```python
from build123d import *

# Parameters (mm, degrees)
SKETCH_1_R          = 4
SKETCH_1_R_2        = 1.5
EXTRUDE_1_DEPTH     = 2
EXTRUDE_2_DEPTH     = 52
EXTRUDE_START       = 2
SKETCH_3_R          = 4
SKETCH_3_R_2        = 1.5
EXTRUDE_3_DEPTH     = 2
FILLET_1_R          = 3
FILLET_2_R          = 1
SKETCH_4_R          = 4
SKETCH_4_R_2        = 1.5
CUT_EXTRUDE_1_DEPTH = 2
SKETCH_5_R          = 1.5
CUT_EXTRUDE_2_DEPTH = 2


with BuildPart() as part:
    # 草图1 → 凸台-拉伸1 (new body)
    with BuildSketch(Plane.XY):
        with BuildLine():
            Line((8.838834765, -8.838834765), (39.597979746, 21.920310217))
            Line((39.597979746, 21.920310217), (4.242640687, 21.920310217))
            Line((4.242640687, 21.920310217), (-8.838834765, 8.838834765))
            ThreePointArc((-8.838834765, 8.838834765), (-8.838834765, -8.838834765), (8.838834765, -8.838834765))
        make_face()
        Circle(SKETCH_1_R, mode=Mode.SUBTRACT)
        with Locations((4.949747468, -4.949747468)):
            Circle(SKETCH_1_R_2, mode=Mode.SUBTRACT)
        with Locations((-4.949747468, -4.949747468)):
            Circle(SKETCH_1_R_2, mode=Mode.SUBTRACT)
        with Locations((-4.949747468, 4.949747468)):
            Circle(SKETCH_1_R_2, mode=Mode.SUBTRACT)
        with Locations((4.949747468, 4.949747468)):
            Circle(SKETCH_1_R_2, mode=Mode.SUBTRACT)
    extrude(amount=EXTRUDE_1_DEPTH)

    # 草图2 → 凸台-拉伸2 (add)
    with BuildSketch(Plane(origin=(0, 0, 0), x_dir=(-1, 0, 0), z_dir=(0, 0, -1))):
        Polygon((-39.597979746, 21.920310217), (-4.242640687, 21.920310217), (-2.242640687, 19.920310217), (-37.597979746, 19.920310217), align=None)
    extrude(amount=EXTRUDE_2_DEPTH)

    # 草图3 → 凸台-拉伸3 (add)
    with BuildSketch(Plane(origin=(0, 0, -52), x_dir=(-1, 0, 0), z_dir=(0, 0, -1)).offset(EXTRUDE_START)):
        with BuildLine():
            Line((-2.242640687, 19.920310217), (-4.242640687, 21.920310217))
            Line((-4.242640687, 21.920310217), (-39.597979746, 21.920310217))
            Line((-39.597979746, 21.920310217), (-37.597979746, 19.920310217))
            Line((-37.597979746, 19.920310217), (-8.838834765, -8.838834765))
            ThreePointArc((-8.838834765, -8.838834765), (8.838834765, -8.838834765), (8.838834765, 8.838834765))
            Line((8.838834765, 8.838834765), (-2.242640687, 19.920310217))
        make_face()
        with Locations(Location((0, 0, 0), (0, 0, 180))):
            Circle(SKETCH_3_R, mode=Mode.SUBTRACT)
        with Locations(Location((-4.949747468, -4.949747468, 0), (0, 0, 180))):
            Circle(SKETCH_3_R_2, mode=Mode.SUBTRACT)
        with Locations(Location((-4.949747468, 4.949747468, 0), (0, 0, 180))):
            Circle(SKETCH_3_R_2, mode=Mode.SUBTRACT)
        with Locations(Location((4.949747468, 4.949747468, 0), (0, 0, 180))):
            Circle(SKETCH_3_R_2, mode=Mode.SUBTRACT)
        with Locations(Location((4.949747468, -4.949747468, 0), (0, 0, 180))):
            Circle(SKETCH_3_R_2, mode=Mode.SUBTRACT)
    extrude(amount=-EXTRUDE_3_DEPTH)

    # 圆角1
    fillet_1_edges = [part.edges().sort_by_distance(p)[0] for p in [
        (21.920310217, 21.920310217, -54),
        (21.920310217, 21.920310217, 2),
    ]]
    fillet(fillet_1_edges, radius=FILLET_1_R)

    # 圆角2
    fillet_2_edges = [part.edges().sort_by_distance(p)[0] for p in [
        (19.920310217, 19.920310217, 0),
        (19.920310217, 19.920310217, -52),
    ]]
    fillet(fillet_2_edges, radius=FILLET_2_R)

    # 草图4 → 切除-拉伸1 (cut)
    with BuildSketch(Plane(origin=(0, 21.920310217, 0), x_dir=(1, 0, 0), z_dir=(0, 1, 0))):
        with Locations(Location((21.920310217, 26, 0), (0, 0, 180))):
            Circle(SKETCH_4_R)
        with Locations(Location((14.920310217, 26, 0), (0, 0, 180))):
            Circle(SKETCH_4_R_2)
        with Locations(Location((21.920310217, 33, 0), (0, 0, 180))):
            Circle(SKETCH_4_R_2)
        with Locations(Location((28.920310217, 26, 0), (0, 0, 180))):
            Circle(SKETCH_4_R_2)
        with Locations(Location((21.920310217, 19, 0), (0, 0, 180))):
            Circle(SKETCH_4_R_2)
    extrude(amount=-CUT_EXTRUDE_1_DEPTH, mode=Mode.SUBTRACT)

    # 草图5 → 切除-拉伸2 (cut)
    with BuildSketch(Plane(origin=(0, 21.920310217, 0), x_dir=(1, 0, 0), z_dir=(0, 1, 0))):
        with Locations(Location((21.920310217, 44.5, 0), (0, 0, 180))):
            Circle(SKETCH_5_R)
        with Locations(Location((21.920310217, 7.5, 0), (0, 0, 180))):
            Circle(SKETCH_5_R)
    extrude(amount=-CUT_EXTRUDE_2_DEPTH, mode=Mode.SUBTRACT)


solid = part.part
```
CAD build for the part. Positions are in the model's coordinates, mm. A direction names the side the tool comes from. Coordinates: 2 decimals unless noted, no trailing zeros. Loops run counter-clockwise (first coordinate to the right, second up) from the corner with the lowest first, then second, coordinate; pieces in that order, holes last. Notation, with made-up numbers: (61, 24) - (68, 24) arc R14 ccw to (68, 30) - close; hole circle Ø6 at (79, -18.75). An arc over 180 degrees is marked (long way). Use CSV: the item, a comma, the result in double quotes. Start each with the question number.
Q1. Probe probe 1 along Z at (x, y) = (-3, -9.5); probe 2 along Y at (x, z) = (23.5, -48); probe 3 along Y at (x, z) = (0, -53.2). List the from-to ranges inside material, lowest first. Write a range as from..to.
Q2. Cut at C-C, the plane y = 0. List the corners of the cut face in (x, z), then the cut area to 3 significant figures.
Q3. Cut at B-B, the plane z = -26. List the corners of the cut face in (x, y), then the cut area to 3 significant figures.
Q4. Cut at A-A, the plane z = -7.5. List the corners of the cut face in (x, y), then the cut area to 3 significant figures.
Q5. Two-plate mould, pull along Z, no slides. Class faces 1 (the cylindrical face through (-0.867, 3.905, -53.014)), 2 (the cylindrical face through (20.15, 21.06, 1.1)), 3 (the cylindrical face through (29.116, 20.934, -24.513)): +Z half, -Z half, draft (parallel to the pull), parting line (faces both ways), or undercut.
Q6. Cut at D-D, the plane x = 29. List the corners of the cut face in (y, z).
Q7. Drop a flat-ended pin along its axis: P1, Ø3.5, axis at x = 14.92, z = -26, coming from the -Y side. Give the stop position or say it passes through.
Q8. 3-axis set-ups, long thin cutter, end or side, ignore diameter. For faces 4 (the flat face through (7, 7, -52)), 5 (the cylindrical face through (22.116, 20.934, -17.513)): which of +Z, -Z, +X, -X, +Y, -Y reach the whole face in a straight line?
Here are the results:
1,probe 1,"-54..-52, 0..2"
1,probe 2,"19.92..21.92"
1,probe 3,"-12.5..-4, 4..17.68"
2,outline,"(-12.5, -54) - (-4, -54) - (-4, -52) - (-12.5, -52) - close; (-12.5, 0) - (-4, 0) - (-4, 2) - (-12.5, 2) - close; (4, -54) - (17.68, -54) - (17.68, -52) - (4, -52) - close; (4, 0) - (17.68, 0) - (17.68, 2) - (4, 2) - close"
2,area,"88.7 mm2"
3,outline,"(2.24, 19.92) - (13.42, 19.92) - (13.42, 21.92) - (4.24, 21.92) - close; (16.42, 19.92) - (17.92, 19.92) - (17.92, 21.92) - (16.42, 21.92) - close; (25.92, 19.92) - (27.42, 19.92) - (27.42, 21.92) - (25.92, 21.92) - close; (30.42, 19.92) - (37.6, 19.92) - (39.6, 21.92) - (30.42, 21.92) - close"
3,area,"42.7 mm2"
4,outline,"(2.24, 19.92) - (20.42, 19.92) - (20.42, 21.92) - (4.24, 21.92) - close; (23.42, 19.92) - (37.6, 19.92) - (39.6, 21.92) - (23.42, 21.92) - close"
4,area,"64.7 mm2"
5,face 1,"draft"
5,face 2,"+Z half"
5,face 3,"undercut"
6,outline,"(11.32, -54) - (18.92, -54) arc R3 ccw to (21.92, -51) - (21.92, -27.5) - (19.92, -27.5) - (19.92, -51) arc R1 cw to (18.92, -52) - (11.32, -52) - close; (11.32, 0) - (18.92, 0) arc R1 cw to (19.92, -1) - (19.92, -24.5) - (21.92, -24.5) - (21.92, -1) arc R3 ccw to (18.92, 2) - (11.32, 2) - close"
7,P1,"y = 19.92"
8,face 4,"+X, -X, -Y"
8,face 5,"+Y, -Y"
